Input: part model. Units: mm. Frame: model coordinates. Face numbers are marked on the shaded views. A direction names the side the tool comes from. Give positions to 0.01 mm unless a question says otherwise; leave off trailing zeros. Loops run counter-clockwise (first coordinate to the right, second up) from the corner with the lowest first, then second, coordinate; pieces in that order, holes last. Notation, with made-up numbers: (47.25, -24.75) -> (73.25, -24.75) arc R13 ccw to (73.25, -3.75) -> close; hole circle Ø7 at (-30.75, 61). An arc over 180 degrees is marked (long way). Answer as a JSON object with one key per item and string values.
```python
from build123d import *

# Parameters (mm, degrees)
BOSS_EXTRUDE1_DEPTH     = 40
CUT_EXTRUDE1_DEPTH      = 4
CUT_EXTRUDE1_DEPTH_BACK = 4
CUT_EXTRUDE1_START      = -20
SKETCH3_R               = 33.884102156
SKETCH3_R_2             = 29.884102156
FILLET1_R               = 2
FILLET2_R               = 2
FILLET3_R               = 2
SKETCH4_R               = 2
CUT_EXTRUDE2_DEPTH      = 7
CHAMFER1_SIZE           = 1.4
FILLET4_R               = 1
FILLET5_R               = 10
FILLET6_R               = 6


with BuildPart() as part:
    # Sketch1 → Boss-Extrude1 (new body)
    with BuildSketch(Plane.XY):
        Polygon((0, 0), (0, 20), (-5, 20), (-5, 0), (-30, 0), (-30, -7), (25, -7), (25, 0), align=None)
    extrude(amount=BOSS_EXTRUDE1_DEPTH)

    # Sketch3 → Cut-Extrude1 (cut, two sides: drawn at the far end of the back side and taken through both)
    with BuildSketch(Plane.XY.offset(40).offset(CUT_EXTRUDE1_START - CUT_EXTRUDE1_DEPTH_BACK)):
        with Locations((5.748786379, 27.884102156)):
            Circle(SKETCH3_R)
        with Locations((5.748786379, 27.884102156)):
            Circle(SKETCH3_R_2, mode=Mode.SUBTRACT)
    extrude(amount=CUT_EXTRUDE1_DEPTH + CUT_EXTRUDE1_DEPTH_BACK, mode=Mode.SUBTRACT)

    # Fillet1
    fillet1_edges = [part.edges().sort_by_distance(p)[0] for p in [
        (-5, 0, 20),
    ]]
    fillet(fillet1_edges, radius=FILLET1_R)

    # Fillet2
    fillet2_edges = [part.edges().sort_by_distance(p)[0] for p in [
        (-5, 20, 20),
    ]]
    fillet(fillet2_edges, radius=FILLET2_R)

    # Fillet3
    fillet3_edges = [part.edges().sort_by_distance(p)[0] for p in [
        (25, 0, 20),
    ]]
    fillet(fillet3_edges, radius=FILLET3_R)

    # Sketch4 → Cut-Extrude2 (cut)
    with BuildSketch(Plane(origin=(0, 0, 0), x_dir=(1, 0, 0), z_dir=(0, 1, 0))):
        with Locations(Location((-24, -6, 0), (0, 0, 180))):
            Circle(SKETCH4_R)
        with Locations(Location((-24, -34, 0), (0, 0, 180))):
            Circle(SKETCH4_R)
        with Locations(Location((19, -34, 0), (0, 0, 180))):
            Circle(SKETCH4_R)
        with Locations(Location((19, -6, 0), (0, 0, 180))):
            Circle(SKETCH4_R)
    extrude(amount=-CUT_EXTRUDE2_DEPTH, mode=Mode.SUBTRACT)

    # Chamfer1
    chamfer1_edges = [part.edges().sort_by_distance(p)[0] for p in [
        (21, 0, 6),
        (21, 0, 34),
        (-22, 0, 34),
        (-22, 0, 6),
    ]]
    chamfer(chamfer1_edges, length=CHAMFER1_SIZE)

    # Fillet4
    fillet4_edges = [part.edges().sort_by_distance(p)[0] for p in [
        (-5, 0, 32),
        (-5, 0, 8),
    ]]
    fillet(fillet4_edges, radius=FILLET4_R)

    # Fillet5
    fillet5_edges = [part.edges().sort_by_distance(p)[0] for p in [
        (0, 0, 20),
    ]]
    fillet(fillet5_edges, radius=FILLET5_R)

    # Fillet6
    fillet6_edges = [part.edges().sort_by_distance(p)[0] for p in [
        (-30, -3.5, 40),
        (25, -3.5, 40),
        (25, -3.5, 0),
        (-30, -3.5, 0),
    ]]
    fillet(fillet6_edges, radius=FILLET6_R)


solid = part.part
```
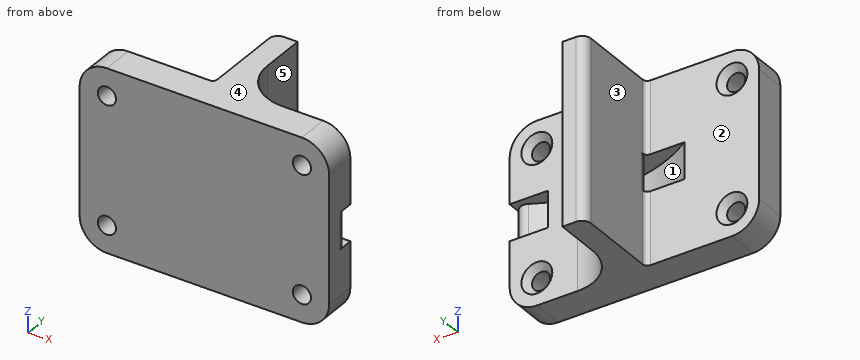
Q1. Section A-A, the plane z = 15. Return the cut outline in (x, y), then the cut area to 3 significant figures.
Evaluation:
{"outline": "(-30, -7) -> (25, -7) -> (25, 0) -> (10, 0) arc R10 cw to (0, 10) -> (0, 20) -> (-3, 20) arc R2 ccw to (-5, 18) -> (-5, 1) arc R1 cw to (-6, 0) -> (-30, 0) -> close", "area": "506 mm2"}
Q2. Section C-C, the plane y = 14.5. Return the cut outline in (x, z), then the cut area to 3 significant figures.
Evaluation:
{"outline": "(-5, 0) -> (0, 0) -> (0, 40) -> (-5, 40) -> close", "area": "200 mm2"}
Q3. Pin query (flat end, axial travel): pin 1 (8.5 mm diameter, centred on y = 7.5, z = 21.5, fed in from -X); pin 2 (12 mm diameter, centred on x = 15, y = 8, fed in from +Z) (3 decimals); pin 3 (5 mm diameter, centred on y = 17, z = 17, fed in from +X); pin 4 (4 mm diameter, centred on y = 3, z = 27.5, fed in from +X). Return the tip coordinate at first contact, or that it passes through.
Evaluation:
{"pin 1": "stops at x = -5", "pin 2": "passes through", "pin 3": "stops at x = 0", "pin 4": "stops at x = 5.64"}
Q4. Section B-B, the plane x = -2. Return the cut outline in (y, z).
Evaluation:
{"outline": "(-7, 0) -> (20, 0) -> (20, 40) -> (-7, 40) -> close; hole (-5.1, 16) -> (-0.98, 16) -> (-0.98, 24) -> (-5.1, 24) -> close"}
Q5. Access query for the marked faces 4 and 5. Directions: +Z, -Z, +X, -X, +Y, -Y. A direction counts if a zero-diameter tool reaches every point of the face in a straight line with its end or side. Return the directions, or none.
Evaluation:
{"face 4": "+Z, +X, -X, +Y, -Y", "face 5": "+Z, -Z, +X, +Y"}
Q6. Section D-D, the plane x = -11. Return the cut outline in (y, z), then the cut area to 3 significant figures.
Evaluation:
{"outline": "(-7, 0) -> (0, 0) -> (0, 16) -> (-1.57, 16) -> (-1.57, 24) -> (0, 24) -> (0, 40) -> (-7, 40) -> close", "area": "267 mm2"}
Q7. Ray query, line 1 along Z through (x, y) = (-24, -5.6); line 2 along Y through (x, z) = (-19, 27); line 3 along Y through (x, z) = (5.5, 18). Return the intervals inside material, ascending.
Evaluation:
{"line 1": "z = 0 to 4, 8 to 32, 36 to 40", "line 2": "y = -7 to 0", "line 3": "y = -7 to -6, -2 to 1.07"}
Q8. Draft query along X for the marked faces 1, 2 and 3. Return one class per face: +X half, -X half, draft (parallel to the pull), parting line (faces both ways), or undercut.
Evaluation:
{"face 1": "undercut", "face 2": "draft", "face 3": "-X half"}
